```python
from build123d import *

# Parameters (mm, degrees)
SKETCH5_R           = 1.6
BOSS_EXTRUDE2_DEPTH = 2
SKETCH6_R           = 6.5
BOSS_EXTRUDE3_DEPTH = 14.5
FILLET1_R           = 1
SKETCH7_R           = 0.5
BOSS_EXTRUDE4_DEPTH = 0.6


with BuildPart() as part:
    # Sketch5 → Boss-Extrude2 (new body)
    with BuildSketch(Plane(origin=(0, 0, 0), x_dir=(1, 0, 0), z_dir=(0, 1, 0))):
        with BuildLine():
            Line((-11.250000051, -22.142785594), (-3.22490315, -22.142785594))
            ThreePointArc((-3.22490315, -22.142785594), (-5.1e-08, -27.342785594), (3.224903048, -22.142785594))
            Line((3.224903048, -22.142785594), (11.249999949, -22.142785594))
            ThreePointArc((11.249999949, -22.142785594), (24.240381006, -14.642785594), (24.240381006, 0.357214406))
            Line((24.240381006, 0.357214406), (20.227832555, 7.30715219))
            ThreePointArc((20.227832555, 7.30715219), (23.118713105, 12.700000199), (17.002929456, 12.892848208))
            Line((17.002929456, 12.892848208), (12.990381006, 19.842785992))
            ThreePointArc((12.990381006, 19.842785992), (-5.1e-08, 27.342785992), (-12.990381108, 19.842785992))
            Line((-12.990381108, 19.842785992), (-17.002929558, 12.892848208))
            ThreePointArc((-17.002929558, 12.892848208), (-23.118713208, 12.700000199), (-20.227832658, 7.30715219))
            Line((-20.227832658, 7.30715219), (-24.240381108, 0.357214406))
            ThreePointArc((-24.240381108, 0.357214406), (-24.240381108, -14.642785594), (-11.250000051, -22.142785594))
        make_face()
        with Locations((20.001021652, 10.900000199)):
            Circle(SKETCH5_R, mode=Mode.SUBTRACT)
        with Locations((-5.1e-08, -23.742785594)):
            Circle(SKETCH5_R, mode=Mode.SUBTRACT)
        with Locations((-20.001021754, 10.900000199)):
            Circle(SKETCH5_R, mode=Mode.SUBTRACT)
    extrude(amount=BOSS_EXTRUDE2_DEPTH)

    # Sketch6 → Boss-Extrude3 (add)
    with BuildSketch(Plane(origin=(0, 0, 0), x_dir=(1, 0, 0), z_dir=(0, 1, 0))):
        with Locations((-0.060025126, 12.462836141)):
            Circle(SKETCH6_R)
        with Locations((11.189974874, -7.022735444)):
            Circle(SKETCH6_R)
        with Locations((-11.310025126, -7.022735444)):
            Circle(SKETCH6_R)
    extrude(amount=BOSS_EXTRUDE3_DEPTH)

    # Fillet1
    fillet1_edges = [part.edges().sort_by_distance(p)[0] for p in [
        (-6.560025126, 14.5, -12.462836141),
        (4.689974874, 14.5, 7.022735444),
        (-17.810025126, 14.5, 7.022735444),
    ]]
    fillet(fillet1_edges, radius=FILLET1_R)

    # Sketch7 → Boss-Extrude4 (add)
    with BuildSketch(Plane(origin=(18.334964129, 0, -10.585696476), x_dir=(-0.5, 0, -0.866025404), z_dir=(0.866025404, 0, -0.5))):
        with Locations((-10.763992659, 1)):
            Circle(SKETCH7_R)
    extrude(amount=BOSS_EXTRUDE4_DEPTH)


solid = part.part
```
For this review, take the finished solid that the model builds, in its own axes (mm). A direction names the side the tool comes from. Give positions to 0.01 mm unless a question says otherwise; leave off trailing zeros. Order: outer loops, then holes, each group sorted by start corner. A loop starts at its lowest first (then second) coordinate and runs counter-clockwise, first axis right, second up.
1) Take a section at A-A (y = 3). Give the boundary of the cut face in (x, z).
2) Insertion check: pin 1 (2 mm diameter, centred on x = -6.5, y = 1, fed in from +Z); pin 2 (1.5 mm diameter, centred on y = 6, z = 11, fed in from +X); pin 3 (3 mm diameter, centred on x = 20, z = -10.9, fed in from -Y); pin 4 (1.5 mm diameter, centred on y = 10.5, z = -7, fed in from -X). Each pin has a flat end and moves straight along its axis. Give the tip position at first contact, or say it passes through.
3) For faces 1 (the face through (24.13, 0.99, 14.83)), 2 (the face through (4.696, 7.67, 6.737)), 3 (the face through (-22.206, 0.986, -3.881)), list the 3-axis set-ups (+Z, -Z, +X, -X, +Y, -Y) from which the entire face can be reached by the end or side of a thin tool; tool diameter is ignored.
4) Take a section at D-D (z = -22). Give the boundary of the cut face in (x, y), then the cut area to 3 significant figures.
5) The part is to be moulded in two halves that separate along Z. For faces 4 (the face through (0, 0, 0)), 5 (the face through (-14.969, 0.986, -16.416)), 6 (the face through (22.262, 0.986, -3.784)), say which applies: released by +Z, released by -Z, zero draft, split by the parting line, or undercut.
6) Take a section at B-B (z = 17.5). Give the boundary of the cut face in (x, y), then the cut area to 3 significant figures.
7) Wall thickness on line 1 (X direction, y = 1.65, z = -10.9); line 2 (Z direction, x = 0, y = 0.9); line 3 (Y direction, x = 20.5, z = 12): over which ranges is each line inside the solid? List them lowest first.
8) Take a section at C-C (z = -10.9). State how many separate pieces and enclosed holes the cut face has, then the cut area to 3 significant figures.
Derived:
1. outline: circle Ø13 at (-11.31, 7.02); circle Ø13 at (-0.06, -12.46); circle Ø13 at (11.19, 7.02)
2. pin 1: stops at z = 22.14
2. pin 2: stops at x = 16.83
2. pin 3: passes through
2. pin 4: stops at x = -4.54
3. face 1: +X, +Y, -Y
3. face 2: +Y
3. face 3: -X, +Y, -Y
4. outline: (-11.48, 0) - (11.48, 0) - (11.48, 2) - (-11.48, 2) - close
4. area: 45.9 mm2
5. face 4: zero draft
5. face 5: released by -Z
5. face 6: undercut
6. outline: (-22.1, 0) - (22.1, 0) - (22.1, 2) - (-22.1, 2) - close
6. area: 88.4 mm2
7. line 1: x = -23.6 to -21.6, -18.4 to 18.4, 21.6 to 23.6
7. line 2: z = -27.34 to 22.14, 25.34 to 27.34
7. line 3: y = 0 to 2
8. separate pieces: 3
8. enclosed holes: 0
8. area: 239 mm2
